Autodesk Inventor part; units mm, degrees
ref_plane "YZ Plane" through (0, 0, 0) normal (1, 0, 0) x (0, 1, 0)
ref_plane "XZ Plane" through (0, 0, 0) normal (0, 1, 0) x (-1, 0, 0)
ref_plane "XY Plane" through (0, 0, 0) normal (0, 0, 1) x (1, 0, 0)
sketch "Skizze1" plane through (0, 0, 0) normal (0, 0, 1) x (1, 0, 0)
  line L0 (-9, 3.5) -> (9, 3.5)
  line L1 (9, 3.5) -> (9, -3.5)
  line L2 (9, -3.5) -> (-9, -3.5)
  line L3 (-9, -3.5) -> (-9, 3.5)
  line L4 (9, -3.5) -> (-9, 3.5) construction
  point P0 (0, 0)
  point P1 (0, 0)
  dimension "d0" = 18
  dimension "d1" = 7
extrude "Extrusion1" add sketch "Skizze1" along normal blind 14
sketch "Skizze2" plane through (0, 0, 14) normal (0, 0, 1) x (1, 0, 0)
  circle A0 centre (-7.5, 0) radius 0.375
  circle A1 centre (7.5, 0) radius 0.375
  line L0 (7.5, 0) -> (-7.5, 0) construction
  point P0 (0, 0)
  point P1 (0, 0)
  dimension "d4" = 15
  dimension "d5" = 0.75
extrude "Extrusion2" add sketch "Skizze2" along normal blind 5
fillet "Rundung1" radius 1.5 4 edges at (9, -3.5, 7) (-9, -3.5, 7) (9, 3.5, 7) (-9, 3.5, 7)
fillet "Rundung2" radius 1.5 8 edges at (-8.5607, -3.0607, 0) (-9, 0, 0) (-8.5607, 3.0607, 0) (0, 3.5, 0) (8.5607, 3.0607, 0) (9, 0, 0) (8.5607, -3.0607, 0) (0, -3.5, 0)
sketch "Skizze3" plane through (-7.5, 0, 19) normal (0, 0, 1) x (1, 0, 0)
  circle A0 centre (0, 0) radius 0.375
  circle A1 centre (15, 0) radius 0.375
  point P0 (7.5, 0)
extrude "Extrusion3" cut sketch "Skizze3" against normal blind 2.5 contours A0
properties part number "MKP4 0,1µF 630VDC (450377)"
Work out the finished part from the listing and answer in its coordinate system (mm). Round coordinates to 2 decimals unless told otherwise and drop trailing zeros. Write each loop counter-clockwise with the first axis right and the second up, starting at its lowest first coordinate (ties: lowest second). Pieces come first, ordered by that corner, then holes. Notation, with made-up numbers: M 16.5,-17.75 L 23.5,-17.75 A26 cw 23.5,17.25 Z; hole C -14.5,-32.75 d6. An arc over 180 degrees is marked long. Use a Markdown table: item, result.
1) The part is cut by section A-A on z = 15.25. Give the vertices of the cut face in (x, y) (3 decimals).
Taken from the geometry:
| item | result |
|---|---|
| outline | C -7.5,0 d0.75; C 7.5,0 d0.75 |
2) Flat-ended cylindrical pins translate along their axes: pin 1 (2 mm diameter, centred on x = 1, y = 0, fed in from +Z); pin 2 (0.8 mm diameter, centred on x = -7.5, y = 0, fed in from +Z). Find the tip coordinate at first contact, or state that the pin passes through.
Taken from the geometry:
| item | result |
|---|---|
| pin 1 | stops at z = 14 |
| pin 2 | stops at z = 16.5 |
3) Consider line 1 (Z direction, x = -4.75, y = 2); line 2 (X direction, y = -3, z = 9); line 3 (X direction, y = -2.5, z = 2). Determine where each line is inside the solid, lowest interval first. Write a range as [from, to].
Taken from the geometry:
| item | result |
|---|---|
| line 1 | z = [0, 14] |
| line 2 | x = [-8.62, 8.62] |
| line 3 | x = [-8.91, 8.91] |
4) The part is cut by section C-C on z = 9.5. Give the vertices of the cut face in (x, y), plus the area to 3 significant figures.
Taken from the geometry:
| item | result |
|---|---|
| outline | M -9,-2 A1.5 ccw -7.5,-3.5 L 7.5,-3.5 A1.5 ccw 9,-2 L 9,2 A1.5 ccw 7.5,3.5 L -7.5,3.5 A1.5 ccw -9,2 Z |
| area | 124 mm2 |
5) The part is cut by section D-D on x = -2.75. Give the vertices of the cut face in (y, z), plus the area to 3 significant figures.
Taken from the geometry:
| item | result |
|---|---|
| outline | M -3.5,1.5 A1.5 ccw -2,0 L 2,0 A1.5 ccw 3.5,1.5 L 3.5,14 L -3.5,14 Z |
| area | 97.0 mm2 |
6) The part is cut by section B-B on y = 1.5. Give the vertices of the cut face in (x, z).
Taken from the geometry:
| item | result |
|---|---|
| outline | M -9,1.5 A1.5 ccw -7.5,0 L 7.5,0 A1.5 ccw 9,1.5 L 9,14 L -9,14 Z |
